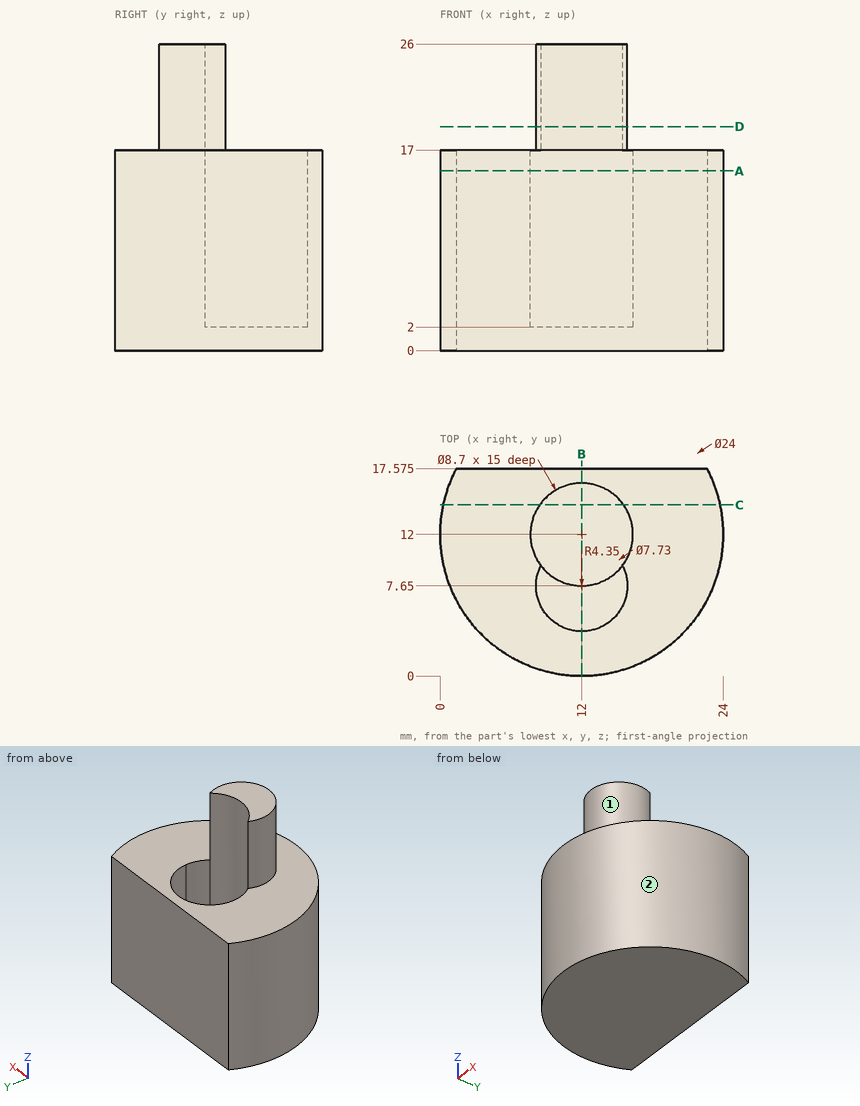
Geometry check sheet. Reference: drawing and pictorial views, mm from the part's lowest x, y, z. A direction names the side the tool comes from. Coordinates: 2 decimals unless noted, no trailing zeros. Order: outer loops, then holes, each group sorted by start corner. A loop starts at its lowest first (then second) coordinate and runs counter-clockwise, first axis right, second up. Notation, with made-up numbers: (89.25, 10) -> (115.25, 10) arc R18 ccw to (115.25, 14) -> close; hole circle Ø8 at (-33, 74.25). An arc over 180 degrees is marked (long way). Use CSV: the item, a comma, the result in double quotes. Start each with the question number.
Q1. Section check A-A, the plane z = 15.25. Record the cut outline in (x, y) (3 decimals).
Q2. Section check C-C, the plane y = 14.5. Record the cut outline in (x, z).
Q3. Thickness scan on line 1 along X through (y, z) = (12, 10.5); line 2 along Z through (x, y) = (14.75, 2); line 3 along X through (y, z) = (15.25, 2.5). Record the ranges inside material, lowest first.
Q4. Tool access check on the marked faces 1 and 2. Record the directions out of +Z, -Z, +X, -X, +Y, -Y that give a thin tool (end or side, any length) a straight path to the whole face; none if there is none.
Q5. Section check B-B, the plane x = 12. Record the cut outline in (y, z) (3 decimals).
Q6. Section check D-D, the plane z = 19. Record the cut outline in (x, y) (3 decimals), and give its area (3 significant figures).
Q7. Depth check by flat-ended pin: P1, Ø1.5, axis at y = 8.5, z = 21.5, coming from the +X side; P2, Ø2, axis at y = 6, z = 22.5, coming from the -X side; P3, Ø3, axis at x = 10, z = 16, coming from the -Y side. Enter the tip coordinate at first touch or a pass-through.
Returned:
1,outline,"(1.374, 17.575) arc R12 ccw (long way) to (22.626, 17.575) -> close; hole circle Ø8.7 at (12, 12)"
2,outline,"(0.26, 0) -> (23.74, 0) -> (23.74, 17) -> (15.56, 17) -> (15.56, 2) -> (8.44, 2) -> (8.44, 17) -> (0.26, 17) -> close"
3,line 1,"x = 0 to 7.65, 16.35 to 24"
3,line 2,"z = 0 to 17"
3,line 3,"x = 0.45 to 9.11, 14.89 to 23.55"
4,face 1,"+Z"
4,face 2,"+Z, -Z"
5,outline,"(0, 0) -> (17.575, 0) -> (17.575, 17) -> (16.35, 17) -> (16.35, 2) -> (7.65, 2) -> (7.65, 26) -> (3.785, 26) -> (3.785, 17) -> (0, 17) -> close"
6,outline,"(8.537, 9.367) arc R3.865 ccw (long way) to (15.463, 9.367) arc R4.35 cw to start"
6,area,"28.0 mm^2"
7,P1,"stops at x = 15.86"
7,P2,"stops at x = 8.19"
7,P3,"stops at y = 0.01"
